For this review, take the finished solid that the model builds, in its own axes (mm). A direction names the side the tool comes from. Round coordinates to 2 decimals unless told otherwise and drop trailing zeros. Order: outer loops, then holes, each group sorted by start corner. A loop starts at its lowest first (then second) coordinate and runs counter-clockwise, first axis right, second up. Notation, with made-up numbers: (5, 71) - (19, 71) arc R21 ccw to (19, 96) - close; hole circle Ø10 at (-37.5, 43.5). An arc over 180 degrees is marked (long way). One line per question, with ' | ' between items.
```python
from build123d import *

# Parameters (mm, degrees)
SKETCH_1_R          = 5.3
SKETCH_1_R_2        = 4.5
EXTRUDE_1_DEPTH     = 0.5
SKETCH_1_4_R        = 7
SKETCH_1_4_R_2      = 5.3
SKETCH_1_4_R_3      = 4.5
EXTRUDE_3_DEPTH     = 3
SKETCH_2_R          = 1.25
SKETCH_2_W          = 2.176030001
SKETCH_2_H          = 2.5
CUT_EXTRUDE_2_DEPTH = 8
SKETCH_3_R          = 7
EXTRUDE_4_DEPTH     = 0.5
SKETCH_4_R          = 3.5
CUT_EXTRUDE_3_DEPTH = 4.5000001
SKETCH_5_W          = 7.173185096
SKETCH_5_H          = 25.447728078
SKETCH_5_W_2        = 11.53458805
SKETCH_5_H_2        = 25.700853956
CUT_EXTRUDE_4_DEPTH = 4.5000001


with BuildPart() as part:
    # Sketch 1 → Extrude 1 (new body)
    with BuildSketch(Plane.XY):
        Circle(SKETCH_1_R)
        Circle(SKETCH_1_R_2, mode=Mode.SUBTRACT)
    extrude(amount=EXTRUDE_1_DEPTH)

    # Sketch 1_4 → Extrude 3 (add)
    with BuildSketch(Plane.XY):
        Circle(SKETCH_1_4_R)
        Circle(SKETCH_1_4_R_2, mode=Mode.SUBTRACT)
        Circle(SKETCH_1_4_R_2)
        Circle(SKETCH_1_4_R_3, mode=Mode.SUBTRACT)
    extrude(amount=-EXTRUDE_3_DEPTH)

    # Sketch 2 → Cut-Extrude 2 (cut, through all)
    with BuildSketch(Plane(origin=(0, 0, 0), x_dir=(0, 0, -1), z_dir=(1, 0, 0))):
        with Locations((1.25, 0)):
            Circle(SKETCH_2_R)
        with Locations((0.161984999, 0)):
            Rectangle(SKETCH_2_W, SKETCH_2_H)
    extrude(amount=-CUT_EXTRUDE_2_DEPTH, mode=Mode.SUBTRACT)

    # Sketch 3 → Extrude 4 (add)
    with BuildSketch(Plane(origin=(0, 0, -3), x_dir=(-1, 0, 0), z_dir=(0, 0, -1))):
        with Locations(Location((0, 0, 0), (0, 0, 180))):  # turned: the seam where the file's is
            Circle(SKETCH_3_R)
    extrude(amount=-EXTRUDE_4_DEPTH)

    # Sketch 4 → Cut-Extrude 3 (cut, through all)
    with BuildSketch(Plane(origin=(0, 0, -3), x_dir=(-1, 0, 0), z_dir=(0, 0, -1))):
        Circle(SKETCH_4_R)
    extrude(amount=-CUT_EXTRUDE_3_DEPTH, mode=Mode.SUBTRACT)

    # Sketch 5 → Cut-Extrude 4 (cut, through all)
    with BuildSketch(Plane(origin=(0, 0, -3), x_dir=(-1, 0, 0), z_dir=(0, 0, -1))):
        with Locations((-9.786592548, -0.021348765)):
            Rectangle(SKETCH_5_W, SKETCH_5_H)
        with Locations((11.967294025, -0.783904042)):
            Rectangle(SKETCH_5_W_2, SKETCH_5_H_2)
    extrude(amount=-CUT_EXTRUDE_4_DEPTH, mode=Mode.SUBTRACT)


solid = part.part
```
(1) We need section B-B on z = -0.4. State the section outline as (x, y) points.
Output values:
outline: (-6.2, -3.25) arc R7 ccw to (6.2, -3.25) - (6.2, 3.25) arc R7 ccw to (-6.2, 3.25) - (-6.2, 1.25) - (-4.32, 1.25) arc R4.5 cw (long way) to (-4.32, -1.25) - (-6.2, -1.25) - close
(2) Insertion check: pin 1 (0.5 mm diameter, centred on x = -5.5, z = 0, fed in from +Y); pin 2 (2 mm diameter, centred on x = 2, z = 0, fed in from -Y); pin 3 (1.5 mm diameter, centred on x = 1.5, z = 0, fed in from -Y). Each pin has a flat end and moves straight along its axis. Give the tip position at first contact, or say it passes through.
Output values:
pin 1: y = 4.63 | pin 2: y = -6.93 | pin 3: y = -6.96
(3) Mouldability with a two-part tool opening along Y and no side actions: class faces 4 (the cylindrical face through (-3.233, -1.341, -2.754)), 5 (the flat face through (4, -3, 0.5)), 6 (the cylindrical face through (5.296, -0.215, 0.246)) as released by +Y, released by -Y, zero draft, split by the parting line, or undercut.
Output values:
face 4: undercut | face 5: zero draft | face 6: split by the parting line
(4) For faces 1 (the flat face through (-5, -1.25, -1)), 2 (the flat face through (5.5, -0.5, 0)), 3 (the cylindrical face through (0, -7, -1)), list the 3-axis set-ups (+Z, -Z, +X, -X, +Y, -Y) from which the entire face can be reached by the end or side of a thin tool; tool diameter is ignored.
Output values:
face 1: +Z, -X | face 2: +Z | face 3: +Z, -Z, -Y
(5) We need section D-D on y = 4.75. State the section outline as (x, z) points, plus the area to 3 significant figures.
Output values:
outline: (-5.14, -3) - (5.14, -3) - (5.14, 0) - (2.35, 0) - (2.35, 0.5) - (-2.35, 0.5) - (-2.35, 0) - (-5.14, 0) - close | area: 33.2 mm^2
(6) For probe 1 along Y at (x, z) = (0, -2.8); probe 2 along Z at (x, y) = (-4, 2); probe 3 along Y at (x, z) = (0.25, -1.5), list the stretches that pass through material, from the lowest coordinate up. Write a range as [from, to].
Output values:
probe 1: [-7, -3.5], [3.5, 7] | probe 2: [-3, -2.5] | probe 3: [-7, -4.49], [4.49, 7]
(7) We need section C-C on y = -1.5. State the section outline as (x, z) points.
Output values:
outline: (-6.2, -3) - (-3.16, -3) - (-3.16, -2.5) - (-4.24, -2.5) - (-4.24, 0.5) - (-5.08, 0.5) - (-5.08, 0) - (-6.2, 0) - close; (3.16, -3) - (6.2, -3) - (6.2, 0) - (5.08, 0) - (5.08, 0.5) - (4.24, 0.5) - (4.24, -2.5) - (3.16, -2.5) - close
(8) We need section A-A on x = 0. State the section outline as (y, z) points.
Output values:
outline: (-7, -3) - (-3.5, -3) - (-3.5, -2.5) - (-4.5, -2.5) - (-4.5, 0.5) - (-5.3, 0.5) - (-5.3, 0) - (-7, 0) - close; (3.5, -3) - (7, -3) - (7, 0) - (5.3, 0) - (5.3, 0.5) - (4.5, 0.5) - (4.5, -2.5) - (3.5, -2.5) - close
